Design review of the part built by this model. Coordinates are the model's own, in mm. Face numbers are marked on the shaded views. A direction names the side the tool comes from. Coordinates: 2 decimals unless noted, no trailing zeros. Loops run counter-clockwise (first coordinate to the right, second up) from the corner with the lowest first, then second, coordinate; pieces in that order, holes last. Notation, with made-up numbers: M -26,32.5 L -18,32.5 A13 cw -18,49.5 Z; hole C 85,34.5 d2. An arc over 180 degrees is marked long. Answer as a JSON object with one key per item and string values. Group by question number.
1. To check wall thickness, follow probe 1 along Y at (x, z) = (0, 1.1); probe 2 along X at (y, z) = (-12, 0.95); probe 3 along Y at (x, z) = (12, 2.5). State the ranges of each line that lie inside material, in increasing order.
2. Machinability: for the marked faces 1 and 2, which of the approach directions +Z, -Z, +X, -X, +Y, -Y give a long, thin tool a straight path to every point of the face, cutting with its end or side? Answer none if there is none.
3. Draft analysis for pull direction X (two halves, no side actions). For the marked faces 3, 4 and 5, state which applies: +X half, -X half, draft (parallel to the pull), parting line (faces both ways), or undercut.
4. Consider section A-A (y = 23.5). State the section outline as (x, z) points, then the cut area to 3 significant figures.
5. Insertion check: pin 1 (2 mm diameter, centred on x = 8.5, z = 3, fed in from -Y); pin 2 (4 mm diameter, centred on x = 0, y = 0, fed in from -Z); pin 3 (2 mm diameter, centred on y = 35, z = 2.5, fed in from -X); pin 4 (0.6 mm diameter, centred on y = 9.5, z = 2, fed in from -X). Each pin has a flat end and moves straight along its axis. Give the tip position at first contact, or say it passes through.
6. Consider section B-B (x = -3.5). State the section outline as (y, z) points.
from build123d import *

# Parameters (mm, degrees)
SKETCH_1_R      = 1.5
EXTRUDE_1_DEPTH = 4
EXTRUDE_START   = -4
SKETCH_2_R      = 1.5
EXTRUDE_2_DEPTH = 4


with BuildPart() as part:
    # Эскиз1 → Бобышка-Вытянуть1 (new body)
    with BuildSketch(Plane.XY):
        with BuildLine():
            ThreePointArc((14.071260881, -6.013492872), (12.319653053, -3.733490841), (9.621977893, -2.738961818))
            ThreePointArc((9.621977893, -2.738961818), (9.902389121, -1.423748614), (10.003874897, -0.082809815))
            ThreePointArc((10.003874897, -0.082809815), (12.872466462, 0.111410875), (15.195472667, 1.805571852))
            ThreePointArc((15.195472667, 1.805571852), (15.146612375, 2.177754087), (15.088637629, 2.548625862))
            ThreePointArc((15.088637629, 2.548625862), (12.382429194, 3.519694937), (9.575317452, 2.897872688))
            ThreePointArc((9.575317452, 2.897872688), (9.100156446, 4.155902197), (8.460565465, 5.338839053))
            ThreePointArc((8.460565465, 5.338839053), (10.768774621, 7.053105583), (11.807079223, 9.734236463))
            ThreePointArc((11.807079223, 9.734236463), (11.564758421, 10.020920215), (11.315478542, 10.301573893))
            ThreePointArc((11.315478542, 10.301573893), (8.513871556, 9.655402442), (6.488561375, 7.614653091))
            ThreePointArc((6.488561375, 7.614653091), (5.408688398, 8.416083426), (4.231086277, 9.065444244))
            ThreePointArc((4.231086277, 9.065444244), (5.246072926, 11.755489103), (4.67002155, 14.572349777))
            ThreePointArc((4.67002155, 14.572349777), (4.311175381, 14.68251498), (3.949734969, 14.783845))
            ThreePointArc((3.949734969, 14.783845), (1.942219856, 12.725587893), (1.341732908, 9.91383494))
            ThreePointArc((1.341732908, 9.91383494), (0, 10.004217632), (-1.341732908, 9.91383494))
            ThreePointArc((-1.341732908, 9.91383494), (-1.942219856, 12.725587893), (-3.949734969, 14.783845))
            ThreePointArc((-3.949734969, 14.783845), (-4.311175381, 14.68251498), (-4.67002155, 14.572349777))
            ThreePointArc((-4.67002155, 14.572349777), (-5.246072926, 11.755489103), (-4.231086277, 9.065444244))
            ThreePointArc((-4.231086277, 9.065444244), (-5.408688398, 8.416083426), (-6.488561375, 7.614653091))
            ThreePointArc((-6.488561375, 7.614653091), (-8.513871556, 9.655402442), (-11.315478542, 10.301573893))
            ThreePointArc((-11.315478542, 10.301573893), (-11.564758421, 10.020920215), (-11.807079223, 9.734236463))
            ThreePointArc((-11.807079223, 9.734236463), (-10.768774621, 7.053105583), (-8.460565465, 5.338839053))
            ThreePointArc((-8.460565465, 5.338839053), (-9.100156446, 4.155902197), (-9.575317452, 2.897872688))
            ThreePointArc((-9.575317452, 2.897872688), (-12.382429194, 3.519694937), (-15.088637629, 2.548625862))
            ThreePointArc((-15.088637629, 2.548625862), (-15.146612375, 2.177754087), (-15.195472667, 1.805571852))
            ThreePointArc((-15.195472667, 1.805571852), (-12.872466462, 0.111410875), (-10.003874897, -0.082809815))
            ThreePointArc((-10.003874897, -0.082809815), (-9.902389121, -1.423748614), (-9.621977893, -2.738961818))
            ThreePointArc((-9.621977893, -2.738961818), (-12.319653053, -3.733490841), (-14.071260881, -6.013492872))
            ThreePointArc((-14.071260881, -6.013492872), (-13.91952392, -6.356833577), (-13.759410906, -6.696349066))
            ThreePointArc((-13.759410906, -6.696349066), (-10.889241154, -6.865655999), (-8.371024733, -5.478167151))
            ThreePointArc((-8.371024733, -5.478167151), (-7.560683217, -6.551369301), (-6.613728339, -7.506195299))
            ThreePointArc((-6.613728339, -7.506195299), (-8.345474114, -9.801319657), (-8.586358225, -12.666370108))
            ThreePointArc((-8.586358225, -12.666370108), (-8.273084972, -12.873171495), (-7.954833402, -13.072226469))
            ThreePointArc((-7.954833402, -13.072226469), (-5.448758719, -11.662925603), (-4.080433364, -9.134245124))
            ThreePointArc((-4.080433364, -9.134245124), (-2.818513813, -9.598976524), (-1.505666768, -9.89026481))
            ThreePointArc((-1.505666768, -9.89026481), (-1.72166611, -12.757298735), (-0.375347502, -15.297764332))
            ThreePointArc((-0.375347502, -15.297764332), (0, -15.302368421), (0.375347502, -15.297764332))
            ThreePointArc((0.375347502, -15.297764332), (1.72166611, -12.757298735), (1.505666768, -9.89026481))
            ThreePointArc((1.505666768, -9.89026481), (2.818513813, -9.598976524), (4.080433364, -9.134245124))
            ThreePointArc((4.080433364, -9.134245124), (5.448758719, -11.662925603), (7.954833402, -13.072226469))
            ThreePointArc((7.954833402, -13.072226469), (8.273084972, -12.873171495), (8.586358225, -12.666370108))
            ThreePointArc((8.586358225, -12.666370108), (8.345474114, -9.801319657), (6.613728339, -7.506195299))
            ThreePointArc((6.613728339, -7.506195299), (7.560683217, -6.551369301), (8.371024733, -5.478167151))
            ThreePointArc((8.371024733, -5.478167151), (10.889241154, -6.865655999), (13.759410906, -6.696349066))
            ThreePointArc((13.759410906, -6.696349066), (13.91952392, -6.356833577), (14.071260881, -6.013492872))
        make_face()
        Circle(SKETCH_1_R, mode=Mode.SUBTRACT)
    extrude(amount=EXTRUDE_1_DEPTH)

    # Эскиз2 → Бобышка-Вытянуть2 (add)
    with BuildSketch(Plane.XY.offset(4).offset(EXTRUDE_START)):
        with BuildLine():
            Line((-7.5, 10.022081122), (-7.5, 0))
            ThreePointArc((-7.5, 0), (0, -7.5), (7.5, 0))
            Line((7.5, 0), (7.5, 14.773393999))
            ThreePointArc((7.5, 14.773393999), (9.729229581, 17.145166049), (10.026172222, 20.386553445))
            Line((10.026172222, 20.386553445), (4.148462459, 44.386107165))
            ThreePointArc((4.148462459, 44.386107165), (3.243079479, 45.620379181), (1.730114922, 45.852938848))
            Line((1.730114922, 45.852938848), (0.876935531, 45.643987428))
            ThreePointArc((0.876935531, 45.643987428), (-0.475250292, 44.512952898), (-0.407285774, 42.751411973))
            ThreePointArc((-0.407285774, 42.751411973), (3.070511892, 30.857094407), (1.383888162, 18.580076554))
            ThreePointArc((1.383888162, 18.580076554), (0.260030802, 16.89805568), (-1.438297092, 15.798996103))
            Line((-1.438297092, 15.798996103), (-4.311175381, 14.68251498))
            ThreePointArc((-4.311175381, 14.68251498), (-6.62649227, 12.84556506), (-7.5, 10.022081122))
        make_face()
        Circle(SKETCH_2_R, mode=Mode.SUBTRACT)
    extrude(amount=EXTRUDE_2_DEPTH)


solid = part.part
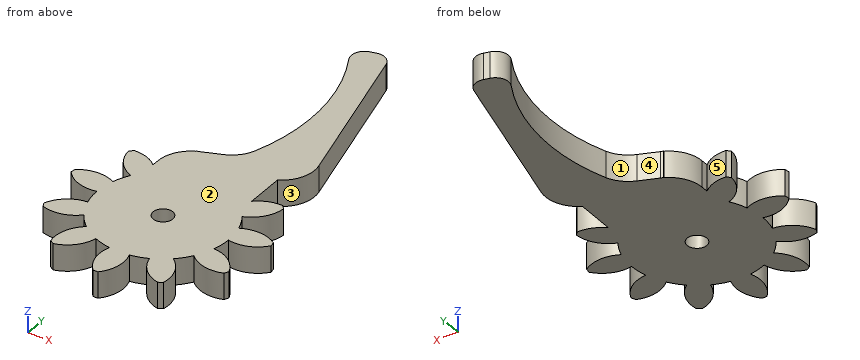
Findings below:
{
 "1": {"probe 1": "y = -15.3 to -1.5, 1.5 to 16.66, 41.97 to 45.17", "probe 2": "x = -8.68 to -5.81, -1.82 to 1.82, 5.81 to 8.68", "probe 3": "y = -6.99 to -3.52, -0.12 to 3.53"},
 "2": {"face 1": "+Z, -Z, -X", "face 2": "+Z, +X, -X, +Y, -Y"},
 "3": {"face 3": "+X half", "face 4": "-X half", "face 5": "undercut"},
 "4": {"outline": "M 2.7,0 L 9.26,0 L 9.26,4 L 2.7,4 Z", "area": "26.3 mm^2"},
 "5": {"pin 1": "stops at y = -13.07", "pin 2": "stops at z = 0", "pin 3": "stops at x = 2.23", "pin 4": "stops at x = -11.81"},
 "6": {"outline": "M -9.37,0 L 15,0 L 15,4 L -9.37,4 Z"}
}
